Part model, mm, in its own coordinate system. Face numbers are marked on the shaded views. A direction names the side the tool comes from. Give positions to 0.01 mm unless a question says otherwise; leave off trailing zeros. Write each loop counter-clockwise with the first axis right and the second up, starting at its lowest first coordinate (ties: lowest second). Pieces come first, ordered by that corner, then holes.
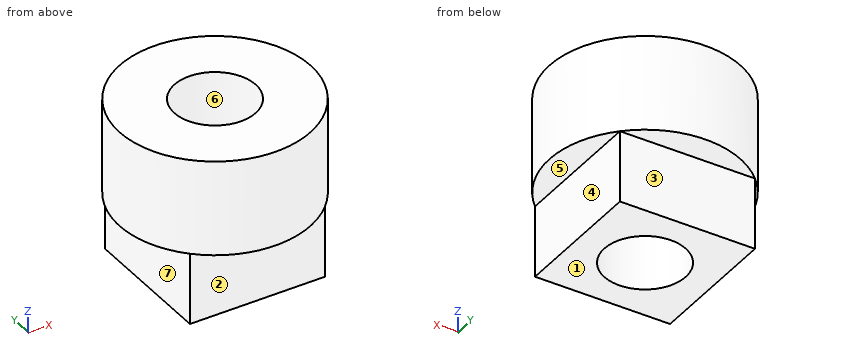
```python
from build123d import *

# Parameters (mm, degrees)
F0_R     = 3.175
F1_DEPTH = 3.175
F2_W     = 4.490128
F2_H     = 4.490128
F3_DEPTH = 2.38125
F4_R     = 1.35255
F5_DEPTH = 6.35


with BuildPart() as f1:
    # F0 (on Top) → F1 (new body)
    with BuildSketch(Plane.XY):
        Circle(F0_R)
    extrude(amount=F1_DEPTH)

    # F2 (on face) → F3 (join)
    with BuildSketch(Plane(origin=(0, 0, 0), x_dir=(1, 0, 0), z_dir=(0, 0, -1))):
        Rectangle(F2_W, F2_H)
    extrude(amount=F3_DEPTH)

    # F4 (on face) → F5 (cut)
    with BuildSketch(Plane(origin=(0, 0, -2.38125), x_dir=(1, 0, 0), z_dir=(0, 0, -1))):
        Circle(F4_R)
    extrude(amount=-F5_DEPTH, mode=Mode.SUBTRACT)


solid = f1.part
```
1) Two-plate mould, pull along X, no slides. Class the marked faces 4, 5, 6 and 7: +X half, -X half, draft (parallel to the pull), parting line (faces both ways), or undercut.
Answers follow:
face 4: +X half
face 5: draft
face 6: undercut
face 7: -X half
2) Saw through at C-C, the plane z = -1. Write the cut outline in (x, y), then the cut area to 3 significant figures.
Answers follow:
outline: (-2.25, -2.25) - (2.25, -2.25) - (2.25, 2.25) - (-2.25, 2.25) - close; hole circle Ø2.71 at (0, 0)
area: 14.4 mm2
3) 3-axis set-ups, long thin cutter, end or side, ignore diameter. For the marked faces 1, 2 and 3: which of +Z, -Z, +X, -X, +Y, -Y reach the whole face in a straight line?
Answers follow:
face 1: -Z, +X, -X, +Y, -Y
face 2: -Z, +X, -X, -Y
face 3: -Z, +X, -X, +Y
4) Wall check: L1, parallel to Y at x = 0, z = -0.2; L2, parallel to X at y = 0, z = 1.2 (3 decimals). Give the ranges that are in metal, low to high.
Answers follow:
L1: y = -2.25 to -1.35, 1.35 to 2.25
L2: x = -3.175 to -1.353, 1.353 to 3.175
5) Saw through at D-D, the plane x = 1.75. Write the cut outline in (y, z) (3 decimals), then the cut area to 3 significant figures.
Answers follow:
outline: (-2.649, 0) - (-2.245, 0) - (-2.245, -2.381) - (2.245, -2.381) - (2.245, 0) - (2.649, 0) - (2.649, 3.175) - (-2.649, 3.175) - close
area: 27.5 mm2
6) Saw through at A-A, the plane y = 0. Write the cut outline in (x, z) (3 decimals).
Answers follow:
outline: (-3.175, 0) - (-2.245, 0) - (-2.245, -2.381) - (-1.353, -2.381) - (-1.353, 3.175) - (-3.175, 3.175) - close; (1.353, -2.381) - (2.245, -2.381) - (2.245, 0) - (3.175, 0) - (3.175, 3.175) - (1.353, 3.175) - close
7) Pin check, flat tips, straight feed: pin 1 Ø2 at (y, z) = (-1, 1) entering from -X (3 decimals); pin 2 Ø2 at (x, y) = (0, 0) entering from -Z; pin 3 Ø1.9 at (x, z) = (-0.5, -1.5) entering from -Y; pin 4 Ø2 at (y, z) = (-0.5, -2) entering from +X. Stop position of each tip, or through.
Answers follow:
pin 1: stops at x = -3.175
pin 2: passes through
pin 3: stops at y = -2.25
pin 4: stops at x = 2.25
